from build123d import *

# Parameters (mm, degrees)
F0_W     = 76.2
F0_H     = 25.4
F1_DEPTH = 9.525
F0_W_2   = 50.8
F2_DEPTH = 15.24
F3_DEPTH = 15.24
F4_DEPTH = 9.525
F6_DEPTH = 1.27
F7_DEPTH = 3.81


with BuildPart() as f1:
    # F0 (on Right) → F1 (new body)
    with BuildSketch(Plane.YZ):
        with Locations((-38.1, 12.7)):
            Rectangle(F0_W, F0_H)
        Polygon((-76.2, -3.175), (-76.2, 0), (-76.2, 25.4), (-101.6, 25.4), (-101.6, -3.175), align=None)
    extrude(amount=F1_DEPTH)

    # F0 (on Right) → F2 (join)
    with BuildSketch(Plane.YZ):
        with Locations((25.4, 12.7)):
            Rectangle(F0_W_2, F0_H)
    extrude(amount=F2_DEPTH)

    # F0 (on Right) → F3 (join)
    with BuildSketch(Plane.YZ):
        with Locations((25.4, 12.7)):
            Rectangle(F0_W_2, F0_H)
    extrude(amount=-F3_DEPTH)

    # F0 (on Right) → F4 (join)
    with BuildSketch(Plane.YZ):
        with Locations((-38.1, 12.7)):
            Rectangle(F0_W, F0_H)
        Polygon((-76.2, -3.175), (-76.2, 0), (-76.2, 25.4), (-101.6, 25.4), (-101.6, -3.175), align=None)
    extrude(amount=-F4_DEPTH)

    # F5 (on face) → F6 (cut)
    with BuildSketch(Plane(origin=(-15.24, 0, 0), x_dir=(0, -1, 0), z_dir=(-1, 0, 0))):
        with BuildLine():
            ThreePointArc((-41.275, 25.4), (-42.204936, 23.154936), (-44.45, 22.225))
            Line((-44.45, 22.225), (-44.45, 12.7))
            Line((-44.45, 12.7), (-42.4688, 12.7))
            Line((-42.4688, 12.7), (-38.8366, 12.7))
            Line((-38.8366, 12.7), (-38.1, 12.7))
            Line((-38.1, 12.7), (-38.1, 25.4))
            Line((-38.1, 25.4), (-41.275, 25.4))
        make_face()
        with BuildLine():
            Line((-38.1, 12.7), (-35.2044, 12.7))
            Line((-35.2044, 12.7), (-31.75, 12.7))
            Line((-31.75, 12.7), (-31.75, 22.225))
            ThreePointArc((-31.75, 22.225), (-33.995064, 23.154936), (-34.925, 25.4))
            Line((-34.925, 25.4), (-38.1, 25.4))
            Line((-38.1, 25.4), (-38.1, 12.7))
        make_face()
        with BuildLine():
            Line((-19.05, 12.7), (-12.7, 12.7))
            Line((-12.7, 12.7), (-12.7, 25.4))
            Line((-12.7, 25.4), (-15.875, 25.4))
            ThreePointArc((-15.875, 25.4), (-16.804936, 23.154936), (-19.05, 22.225))
            Line((-19.05, 22.225), (-19.05, 12.7))
        make_face()
        with BuildLine():
            Line((-6.35, 12.7), (-6.35, 22.225))
            ThreePointArc((-6.35, 22.225), (-8.595064, 23.154936), (-9.525, 25.4))
            Line((-9.525, 25.4), (-12.7, 25.4))
            Line((-12.7, 25.4), (-12.7, 12.7))
            Line((-12.7, 12.7), (-6.35, 12.7))
        make_face()
    extrude(amount=-F6_DEPTH, mode=Mode.SUBTRACT)

    # F5 (on face) → F7 (cut)
    with BuildSketch(Plane(origin=(-15.24, 0, 0), x_dir=(0, -1, 0), z_dir=(-1, 0, 0))):
        with BuildLine():
            Line((-44.45, 25.4), (-47.625, 25.4))
            ThreePointArc((-47.625, 25.4), (-46.695064, 23.154936), (-44.45, 22.225))
            Line((-44.45, 22.225), (-44.45, 25.4))
        make_face()
        with BuildLine():
            Line((-41.275, 25.4), (-44.45, 25.4))
            Line((-44.45, 25.4), (-44.45, 22.225))
            ThreePointArc((-44.45, 22.225), (-42.204936, 23.154936), (-41.275, 25.4))
        make_face()
        with BuildLine():
            ThreePointArc((-34.925, 25.4), (-33.995064, 23.154936), (-31.75, 22.225))
            Line((-31.75, 22.225), (-31.75, 25.4))
            Line((-31.75, 25.4), (-34.925, 25.4))
        make_face()
        with BuildLine():
            ThreePointArc((-31.75, 22.225), (-29.504936, 23.154936), (-28.575, 25.4))
            Line((-28.575, 25.4), (-31.75, 25.4))
            Line((-31.75, 25.4), (-31.75, 22.225))
        make_face()
        with BuildLine():
            ThreePointArc((-22.225, 25.4), (-21.295064, 23.154936), (-19.05, 22.225))
            Line((-19.05, 22.225), (-19.05, 25.4))
            Line((-19.05, 25.4), (-22.225, 25.4))
        make_face()
        with BuildLine():
            ThreePointArc((-19.05, 22.225), (-16.804936, 23.154936), (-15.875, 25.4))
            Line((-15.875, 25.4), (-19.05, 25.4))
            Line((-19.05, 25.4), (-19.05, 22.225))
        make_face()
        with BuildLine():
            Line((-6.35, 22.225), (-6.35, 25.4))
            Line((-6.35, 25.4), (-9.525, 25.4))
            ThreePointArc((-9.525, 25.4), (-8.595064, 23.154936), (-6.35, 22.225))
        make_face()
        with BuildLine():
            ThreePointArc((-6.35, 22.225), (-4.104936, 23.154936), (-3.175, 25.4))
            Line((-3.175, 25.4), (-6.35, 25.4))
            Line((-6.35, 25.4), (-6.35, 22.225))
        make_face()
    extrude(amount=-F7_DEPTH, mode=Mode.SUBTRACT)


solid = f1.part
Verification items for the finished model (mm, model axes). A direction names the side the tool comes from. Coordinates: 2 decimals unless noted, no trailing zeros. Write each loop counter-clockwise with the first axis right and the second up, starting at its lowest first coordinate (ties: lowest second). Pieces come first, ordered by that corner, then holes. Notation, with made-up numbers: (42.25, 54.5) -> (48.25, 54.5) arc R25 ccw to (48.25, 84.5) -> close; hole circle Ø3 at (47, -32). An arc over 180 degrees is marked (long way). One line per item, written item: value. Start each with the question number.
Q1. Cross-section at A-A on z = 16. Enter the section's corners in (x, y) (3 decimals).
Q2. Thickness scan on L1, parallel to Z at x = 11, y = 33.5; L2, parallel to X at y = -67, z = 23.25 (3 decimals); L3, parallel to Y at x = -10, z = 21.5. Record the ranges inside material, lowest first. Write a range as from..to.
Q3. Cross-section at B-B on x = 1.5. Enter the section's corners in (y, z) (3 decimals), and give its area (3 significant figures).
Q4. Mould release check, pull along Y, two halves, no side actions. Record for faces 4 (the flat face through (0, -76.2, -2)), 5 (the flat face through (0, -101.6, 11)), 6 (the flat face through (-9.525, -52, 11)), 7 (the flat face through (-13.97, 38, 19)): pulls with the +Y half, pulls with the -Y half, needs draft (parallel to the pull), parting line crosses it, or undercut.
Q5. Cross-section at C-C on y = -35.5. Enter the section's corners in (x, z) (3 decimals).
Q6. Access from +Z, -Z, +X, -X, +Y, -Y to the whole of each face (thin tool, end or side, straight path). Record for faces 1 (the flat face through (12, 0, 13)), 2 (the flat face through (0, 1, 0)), 3 (the flat face through (-11.43, 44, 24)).
Q7. Go/stop test with flat-tipped pins: P1, Ø1, axis at y = 5, z = 24.5, coming from the -X side; P2, Ø0.6, axis at x = -14.5, z = 17.5, coming from the -Y side; P3, Ø1, axis at y = -32.5, z = 21, coming from the +X side (3 decimals). Record where each tip stops, or that it passes through.
Q8. Cross-section at D-D on z = 5. Enter the section's corners in (x, y) (3 decimals).
Checked values:
1. outline: (-15.24, 0) -> (-9.525, 0) -> (-9.525, -101.6) -> (9.525, -101.6) -> (9.525, 0) -> (15.24, 0) -> (15.24, 50.8) -> (-15.24, 50.8) -> (-15.24, 44.45) -> (-13.97, 44.45) -> (-13.97, 31.75) -> (-15.24, 31.75) -> (-15.24, 19.05) -> (-13.97, 19.05) -> (-13.97, 6.35) -> (-15.24, 6.35) -> close
2. L1: z = 0..25.4
2. L2: x = -9.525..9.525
2. L3: y = 0..50.8
3. outline: (-101.6, -3.175) -> (-76.2, -3.175) -> (-76.2, 0) -> (50.8, 0) -> (50.8, 25.4) -> (-101.6, 25.4) -> close
3. area: 3,950 mm²
4. face 4: pulls with the +Y half
4. face 5: pulls with the -Y half
4. face 6: needs draft
4. face 7: undercut
5. outline: (-9.525, 0) -> (9.525, 0) -> (9.525, 25.4) -> (-9.525, 25.4) -> close
6. face 1: +Z, -Z, +X, -Y
6. face 2: -Z, +X, -X, +Y
6. face 3: +Z, -X
7. P1: stops at x = -11.43
7. P2: stops at y = 0
7. P3: stops at x = 9.525
8. outline: (-15.24, 0) -> (-9.525, 0) -> (-9.525, -101.6) -> (9.525, -101.6) -> (9.525, 0) -> (15.24, 0) -> (15.24, 50.8) -> (-15.24, 50.8) -> close
